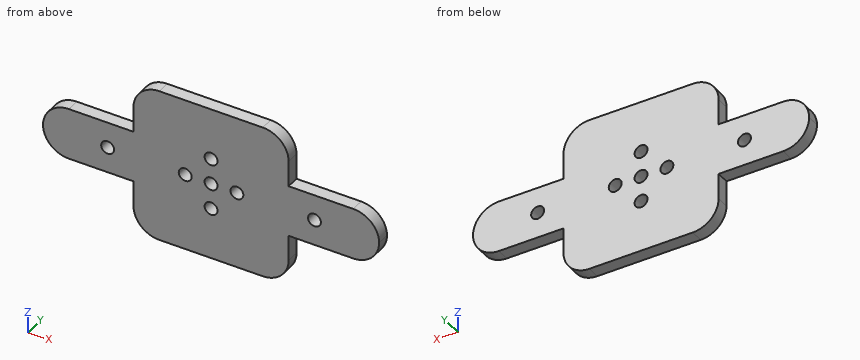
from build123d import *

# Parameters (mm, degrees)
SKETCH1_W           = 60
SKETCH1_H           = 60
SKETCH1_R           = 2.5
BOSS_EXTRUDE2_DEPTH = 5
SKETCH3_W           = 35
SKETCH3_H           = 20
BOSS_EXTRUDE3_DEPTH = 5
SKETCH5_R           = 2.5
CUT_EXTRUDE1_DEPTH  = 113.472218792
FILLET1_R           = 10
FILLET2_R           = 10
FILLET3_R           = 10


with BuildPart() as part:
    # Sketch1 → Boss-Extrude2 (new body)
    with BuildSketch(Plane(origin=(0, 0, 0), x_dir=(1, 0, 0), z_dir=(0, 1, 0))):
        with Locations((30, 30)):
            Rectangle(SKETCH1_W, SKETCH1_H)
        with Locations(Location((30, 40.020691429, 0), (0, 0, 270))):
            Circle(SKETCH1_R, mode=Mode.SUBTRACT)
        with Locations(Location((20, 30.020691429, 0), (0, 0, 270))):
            Circle(SKETCH1_R, mode=Mode.SUBTRACT)
        with Locations(Location((30, 20.020691429, 0), (0, 0, 270))):
            Circle(SKETCH1_R, mode=Mode.SUBTRACT)
        with Locations(Location((40, 30.020691429, 0), (0, 0, 270))):
            Circle(SKETCH1_R, mode=Mode.SUBTRACT)
        with Locations(Location((30, 30.020691429, 0), (0, 0, 270))):
            Circle(SKETCH1_R, mode=Mode.SUBTRACT)
    extrude(amount=BOSS_EXTRUDE2_DEPTH)

    # Sketch3 → Boss-Extrude3 (add)
    with BuildSketch(Plane(origin=(0, 0, 0), x_dir=(1, 0, 0), z_dir=(0, 1, 0))):
        with Locations((77.5, 30.020691429)):
            Rectangle(SKETCH3_W, SKETCH3_H)
        with Locations((-17.5, 30.020691429)):
            Rectangle(SKETCH3_W, SKETCH3_H)
    extrude(amount=BOSS_EXTRUDE3_DEPTH)

    # Sketch5 → Cut-Extrude1 (cut, through all)
    with BuildSketch(Plane(origin=(0, 0, 0), x_dir=(1, 0, 0), z_dir=(0, 1, 0))):
        with Locations(Location((70, 30.020691429, 0), (0, 0, 270))):
            Circle(SKETCH5_R)
        with Locations(Location((-10, 30.020691429, 0), (0, 0, 270))):
            Circle(SKETCH5_R)
    extrude(amount=CUT_EXTRUDE1_DEPTH, mode=Mode.SUBTRACT)

    # Fillet1
    fillet1_edges = [part.edges().sort_by_distance(p)[0] for p in [
        (95, 2.5, -20.020691429),
        (95, 2.5, -40.020691429),
    ]]
    fillet(fillet1_edges, radius=FILLET1_R - 0.0001)  # a hair under: the kernel refuses the full size

    # Fillet2
    fillet2_edges = [part.edges().sort_by_distance(p)[0] for p in [
        (-35, 2.5, -20.020691429),
        (-35, 2.5, -40.020691429),
    ]]
    fillet(fillet2_edges, radius=FILLET2_R - 0.0001)  # a hair under: the kernel refuses the full size

    # Fillet3
    fillet3_edges = [part.edges().sort_by_distance(p)[0] for p in [
        (0, 2.5, -60),
        (60, 2.5, -60),
        (60, 2.5, 0),
        (0, 2.5, 0),
    ]]
    fillet(fillet3_edges, radius=FILLET3_R)


solid = part.part
Geometry: final body of the model. Coordinates: model frame, mm. Round coordinates to 2 decimals unless told otherwise and drop trailing zeros. Order: outer loops, then holes, each group sorted by start corner. A loop starts at its lowest first (then second) coordinate and runs counter-clockwise, first axis right, second up. Notation, with made-up numbers: (34.25, -27) - (61.25, -27) arc R10 ccw to (61.25, -14) - close; hole circle Ø5 at (-5.5, -14.5). An arc over 180 degrees is marked (long way). Write each question's results on one line, items separated by ' | '.
Item 1: Section D-D, the plane z = -16. Return the cut outline in (x, y), and give its area (3 significant figures).
Completed:
outline: (0, 0) - (60, 0) - (60, 5) - (0, 5) - close | area: 300 mm^2
Item 2: Section C-C, the plane x = 70. Return the cut outline in (y, z), and give its area (3 significant figures).
Completed:
outline: (0, -40.02) - (5, -40.02) - (5, -32.52) - (0, -32.52) - close; (0, -27.52) - (5, -27.52) - (5, -20.02) - (0, -20.02) - close | area: 75.0 mm^2
Item 3: Section B-B, the plane y = 1.8. State how many separate pieces and enclosed holes the cut face has, and give its area (3 significant figures).
Completed:
separate pieces: 1 | enclosed holes: 7 | area: 4,690 mm^2
Item 4: Material intervals for line 1 along X through (y, z) = (3.95, -31); line 2 along X through (y, z) = (4.1, -9.5); line 3 along Z through (x, y) = (63.5, 2.1), sorted ascending. Write a range as [from, to].
Completed:
line 1: [-34.95, -12.3], [-7.7, 17.7], [22.3, 27.7], [32.3, 37.7], [42.3, 67.7], [72.3, 94.95] | line 2: [0.01, 59.99] | line 3: [-40.02, -20.02]
Item 5: First-contact query: pin 1 Ø1.5 at (y, z) = (2.5, -15.5) entering from -X; pin 2 Ø2.5 at (x, y) = (-13.5, 3) entering from +Z; pin 3 Ø1.5 at (x, y) = (76.5, 3) entering from -Z. Flat tips, straight axial feed; report the tip coordinate or a pass-through.
Completed:
pin 1: x = 0 | pin 2: z = -20.02 | pin 3: z = -40.02
Item 6: Section A-A, the plane x = 40. Return the cut outline in (y, z), and give its area (3 significant figures).
Completed:
outline: (0, -60) - (5, -60) - (5, -32.52) - (0, -32.52) - close; (0, -27.52) - (5, -27.52) - (5, 0) - (0, 0) - close | area: 275 mm^2
